Part model, mm, in its own coordinate system. A direction names the side the tool comes from. Round coordinates to 2 decimals unless told otherwise and drop trailing zeros. Loops run counter-clockwise (first coordinate to the right, second up) from the corner with the lowest first, then second, coordinate; pieces in that order, holes last. Notation, with made-up numbers: M -20,21.5 L 25,21.5 A32 cw 25,52.5 Z; hole C -15.5,9 d1. An arc over 180 degrees is marked long. Write each question's results on one line, items separated by ' | '.
from build123d import *

# Parameters (mm, degrees)
F0_W     = 105
F0_H     = 146.5
F0_R     = 1.75
F1_DEPTH = 3
F2_W     = 81.692316
F2_H     = 127.184674
F3_DEPTH = 25
F4_R     = 5


with BuildPart() as f1:
    # F0 (on Top) → F1 (new body)
    with BuildSketch(Plane.XY):
        Rectangle(F0_W, F0_H)
        with Locations((-47.5, -69.25)):
            Circle(F0_R, mode=Mode.SUBTRACT)
        with Locations((-48.26, -47.625)):
            Circle(F0_R, mode=Mode.SUBTRACT)
        with Locations((47.5, -69.25)):
            Circle(F0_R, mode=Mode.SUBTRACT)
        with Locations((48.26, -47.625)):
            Circle(F0_R, mode=Mode.SUBTRACT)
        with Locations((-48.26, 47.625)):
            Circle(F0_R, mode=Mode.SUBTRACT)
        with Locations((-47.5, 69.25)):
            Circle(F0_R, mode=Mode.SUBTRACT)
        with Locations((48.26, 47.625)):
            Circle(F0_R, mode=Mode.SUBTRACT)
        with Locations((47.5, 69.25)):
            Circle(F0_R, mode=Mode.SUBTRACT)
    extrude(amount=F1_DEPTH)

    # F2 (on face) → F3 (cut)
    with BuildSketch(Plane.XY.offset(3)):
        Rectangle(F2_W, F2_H)
    extrude(amount=-F3_DEPTH, mode=Mode.SUBTRACT)

    # F4
    f4_edges = [f1.edges().sort_by_distance(p)[0] for p in [
        (-52.5, 73.25, 1.5),
        (-52.5, -73.25, 1.5),
        (52.5, -73.25, 1.5),
        (-40.846158, 63.592337, 1.5),
        (52.5, 73.25, 1.5),
        (40.846158, 63.592337, 1.5),
        (40.846158, -63.592337, 1.5),
        (-40.846158, -63.592337, 1.5),
    ]]
    fillet(f4_edges, radius=F4_R)


solid = f1.part
Item 1: Two-plate mould, pull along X, no slides. Class faces 1 (the cylindrical face through (51, 71.82, 1.52)), 2 (the cylindrical face through (39.34, -62.17, 1.48)), 3 (the cylindrical face through (-51.07, -71.75, 1.52)), 4 (the cylindrical face through (39.42, 62.09, 1.48)): +X half, -X half, draft (parallel to the pull), parting line (faces both ways), or undercut.
Filled sheet:
face 1: +X half | face 2: undercut | face 3: -X half | face 4: undercut
Item 2: Wall check: L1, parallel to Y at x = 10.5, z = 2.05; L2, parallel to X at y = -37.5, z = 1.5; L3, parallel to X at y = 69.25, z = 2.15. Give the ranges that are in metal, low to high.
Filled sheet:
L1: -73.25 to -63.59, 63.59 to 73.25 | L2: -52.5 to -40.85, 40.85 to 52.5 | L3: -52.4 to -49.25, -45.75 to 45.75, 49.25 to 52.4
Item 3: Which spindle directions (+Z, -Z, +X, -X, +Y, -Y) get a long thin tool onto all of the face, cutting with end or side? Do faces 5 (the flat face through (46, 1, 3)), 6 (the flat face through (40.846, -1, 2)). Say none if no direction does.
Filled sheet:
face 5: +Z, +X, -X, +Y, -Y | face 6: +Z, -Z
Item 4: Band-saw the part on B-B on x = -2.5. Give the cut face in (y, z), and give its area (3 significant figures).
Filled sheet:
outline: M -73.25,0 L -63.59,0 L -63.59,3 L -73.25,3 Z; M 63.59,0 L 73.25,0 L 73.25,3 L 63.59,3 Z | area: 57.9 mm^2
Item 5: Drop a flat-ended pin along its axis: P1, Ø5.5, axis at x = -48.26, y = -47.625, coming from the -Z side. Give the stop position or say it passes through.
Filled sheet:
P1: z = 0
Item 6: Band-saw the part on A-A on y = -57. Give the cut face in (x, z), and give its area (3 significant figures).
Filled sheet:
outline: M -52.5,0 L -40.85,0 L -40.85,3 L -52.5,3 Z; M 40.85,0 L 52.5,0 L 52.5,3 L 40.85,3 Z | area: 69.9 mm^2
Item 7: Band-saw the part on C-C on z = 1.25. Count the separate pieces of the cut face and the enclosed holes in it, and give its area (3 significant figures).
Filled sheet:
separate pieces: 1 | enclosed holes: 9 | area: 4,920 mm^2
